Build history of the part. All positions in model axes, mm. Round coordinates to 2 decimals unless told otherwise and drop trailing zeros. Loops run counter-clockwise (first coordinate to the right, second up) from the corner with the lowest first, then second, coordinate; pieces in that order, holes last. Notation, with made-up numbers: (53.5, 25) - (89.5, 25) arc R22 cw to (89.5, 57) - close; hole circle Ø3 at (15.5, 27.25). An arc over 180 degrees is marked (long way). Use a Markdown table: item, result.
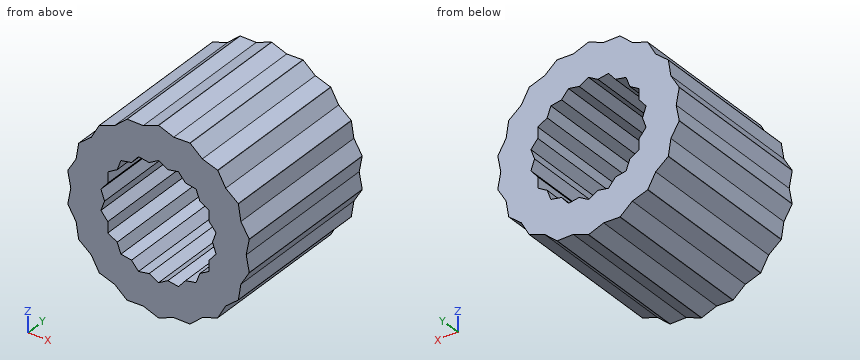
from build123d import *

# Parameters (mm, degrees)
BOSS_EXTRUDE1_DEPTH = 7
SKETCH2_R           = 5.515074568
SKETCH2_R_2         = 4.096991853
CUT_EXTRUDE1_DEPTH  = 10


with BuildPart() as part:
    # Sketch1 → Boss-Extrude1 (new body)
    with BuildSketch(Plane(origin=(0, 0, 0), x_dir=(1, 0, 0), z_dir=(0, 1, 0))):
        Polygon((0, 4.1), (-0.677227893, 3.840750237), (-1.402282588, 3.852739745), (-1.95, 3.377499075), (-2.6354292, 3.140782217), (-2.987573328, 2.506871678), (-3.550704156, 2.05), (-3.664801221, 1.333878559), (-4.037711787, 0.711957528), (-3.9, 0), (-4.037711787, -0.711957528), (-3.664801221, -1.333878559), (-3.550704156, -2.05), (-2.987573328, -2.506871678), (-2.6354292, -3.140782217), (-1.95, -3.377499075), (-1.402282588, -3.852739745), (-0.677227893, -3.840750237), (0, -4.1), (0.677227893, -3.840750237), (1.402282588, -3.852739745), (1.95, -3.377499075), (2.6354292, -3.140782217), (2.987573328, -2.506871678), (3.550704156, -2.05), (3.664801221, -1.333878559), (4.037711787, -0.711957528), (3.9, 0), (4.037711787, 0.711957528), (3.664801221, 1.333878559), (3.550704156, 2.05), (2.987573328, 2.506871678), (2.6354292, 3.140782217), (1.95, 3.377499075), (1.402282588, 3.852739745), (0.677227893, 3.840750237), align=None)
        Polygon((0, 2.6), (-0.416755626, 2.363538607), (-0.889252373, 2.443200814), (-1.2, 2.078460969), (-1.671247785, 1.991715552), (-1.838506663, 1.542690263), (-2.25166605, 1.3), (-2.25526229, 0.820848344), (-2.560500158, 0.451485262), (-2.4, 0), (-2.560500158, -0.451485262), (-2.25526229, -0.820848344), (-2.25166605, -1.3), (-1.838506663, -1.542690263), (-1.671247785, -1.991715552), (-1.2, -2.078460969), (-0.889252373, -2.443200814), (-0.416755626, -2.363538607), (0, -2.6), (0.416755626, -2.363538607), (0.889252373, -2.443200814), (1.2, -2.078460969), (1.671247785, -1.991715552), (1.838506663, -1.542690263), (2.25166605, -1.3), (2.25526229, -0.820848344), (2.560500158, -0.451485262), (2.4, 0), (2.560500158, 0.451485262), (2.25526229, 0.820848344), (2.25166605, 1.3), (1.838506663, 1.542690263), (1.671247785, 1.991715552), (1.2, 2.078460969), (0.889252373, 2.443200814), (0.416755626, 2.363538607), align=None, mode=Mode.SUBTRACT)
    extrude(amount=BOSS_EXTRUDE1_DEPTH)

    # Sketch2 → Cut-Extrude1 (cut)
    with BuildSketch(Plane(origin=(0, 7, 0), x_dir=(1, 0, 0), z_dir=(0, 1, 0))):
        Circle(SKETCH2_R)
        Circle(SKETCH2_R_2, mode=Mode.SUBTRACT)
    extrude(amount=-CUT_EXTRUDE1_DEPTH, mode=Mode.SUBTRACT)


solid = part.part
Q1. Probe line 1 (Z direction, x = -0.75, y = 0.5); line 2 (X direction, y = 4, z = -0.75); line 3 (X direction, y = 6.75, z = 0.25). List the from-to ranges inside material, lowest first.
Results found:
| item | result |
|---|---|
| line 1 | z = -3.84 to -2.42, 2.42 to 3.84 |
| line 2 | x = -4.01 to -2.31, 2.31 to 4.01 |
| line 3 | x = -3.95 to -2.49, 2.49 to 3.95 |
Q2. Drop flat-ended pins along their axis: pin 1 (4 mm diameter, centred on y = 1, z = 3, fed in from +X) (3 decimals); pin 2 (1 mm diameter, centred on y = 1, z = -2, fed in from +X); pin 3 (1.5 mm diameter, centred on y = 4.5, z = 3, fed in from -X). Give the stop position or say it passes through.
Results found:
| item | result |
|---|---|
| pin 1 | stops at x = 3.865 |
| pin 2 | stops at x = 3.64 |
| pin 3 | stops at x = -3.3 |
Q3. Cut at D-D, the plane x = 3.25. List the corners of the cut face in (y, z).
Results found:
| item | result |
|---|---|
| outline | (0, -2.29) - (7, -2.29) - (7, 2.29) - (0, 2.29) - close |
Q4. Cut at A-A, the plane x = 0.25. List the corners of the cut face in (y, z), plus the area to 3 significant figures.
Results found:
| item | result |
|---|---|
| outline | (0, -4) - (7, -4) - (7, -2.46) - (0, -2.46) - close; (0, 2.46) - (7, 2.46) - (7, 4) - (0, 4) - close |
| area | 21.6 mm2 |
Q5. Cut at B-B, the plane z = 1. List the corners of the cut face in (x, y) (3 decimals), plus the area to 3 significant figures.
Results found:
| item | result |
|---|---|
| outline | (-3.865, 0) - (-2.254, 0) - (-2.254, 7) - (-3.865, 7) - close; (2.254, 0) - (3.865, 0) - (3.865, 7) - (2.254, 7) - close |
| area | 22.6 mm2 |
Q6. Cut at C-C, the plane z = -3.5. List the corners of the cut face in (x, y).
Results found:
| item | result |
|---|---|
| outline | (-1.81, 0) - (1.81, 0) - (1.81, 7) - (-1.81, 7) - close |
